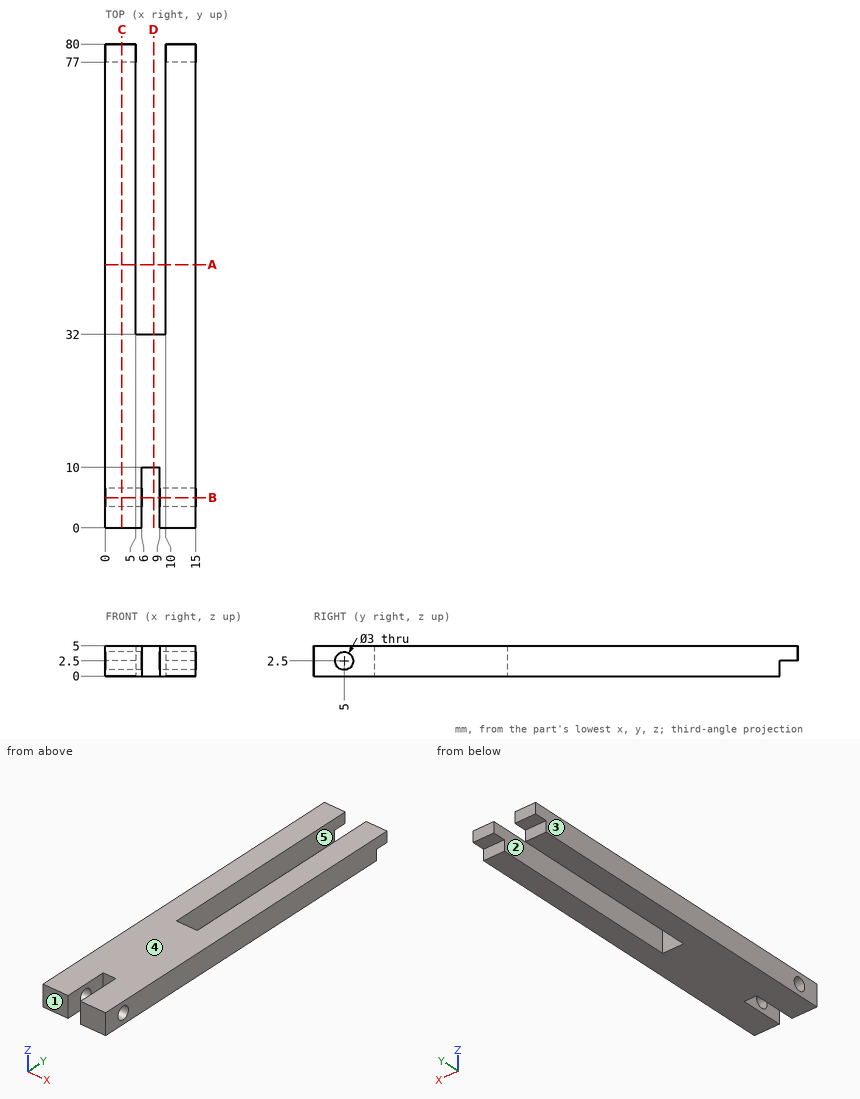
The drawing under review shows one solid part. Ordinate dimensions are in mm from its lowest x, y, z. A direction names the side the tool comes from. Coordinates: 2 decimals unless noted, no trailing zeros. Loops run counter-clockwise (first coordinate to the right, second up) from the corner with the lowest first, then second, coordinate; pieces in that order, holes last. Notation, with made-up numbers: M 23,47.5 L 66,47.5 A8 cw 66,53.5 Z; hole C -11,45 d9. An arc over 180 degrees is marked long. Use one line per item in the form item = value.
(1) Clearance check with flat-ended pins moving along their axes: P1, Ø1.5, axis at x = 13, y = 79, coming from the -Z side; P2, Ø2.5, axis at x = 7.5, z = 1.5, coming from the -Y side; P3, Ø0.8, axis at x = 3, z = 1, coming from the +Y side; P4, Ø1.8, axis at y = 5, z = 2.5, coming from the +X side. State where each tip first meets the part, or that it passes through.
Return value:
P1 = 2.5
P2 = 10
P3 = 77
P4 = through
(2) Consider section D-D (x = 8). Write out the cut boundary in (y, z), and give its area (3 significant figures).
Return value:
outline = M 10,0 L 32,0 L 32,5 L 10,5 Z
area = 110 mm2
(3) Draft analysis for pull direction X (two halves, no side actions). For the marked faces 3, 4 and 5, state which applies: pulls with the +X half, pulls with the -X half, needs draft (parallel to the pull), parting line crosses it, or undercut.
Return value:
face_3 = pulls with the -X half
face_4 = needs draft
face_5 = undercut
(4) Consider section C-C (x = 2.75). Write out the cut boundary in (y, z).
Return value:
outline = M 0,0 L 77,0 L 77,2.5 L 80,2.5 L 80,5 L 0,5 Z; hole C 5,2.5 d3
(5) Consider section A-A (y = 43.5). Write out the cut boundary in (x, z).
Return value:
outline = M 0,0 L 5,0 L 5,5 L 0,5 Z; M 10,0 L 15,0 L 15,5 L 10,5 Z
(6) Consider section B-B (y = 5). Write out the cut boundary in (x, z).
Return value:
outline = M 0,0 L 6,0 L 6,1 L 0,1 Z; M 0,4 L 6,4 L 6,5 L 0,5 Z; M 9,0 L 15,0 L 15,1 L 9,1 Z; M 9,4 L 15,4 L 15,5 L 9,5 Z
(7) For the marked faces 1 and 2, list the 3-axis set-ups (+Z, -Z, +X, -X, +Y, -Y) from which the entire face can be reached by the end or side of a thin tool; tool diameter is ignored.
Return value:
face_1 = +Z, -Z, +X, -X, -Y
face_2 = +Z, -Z, +Y
(8) For line 1 along X through (y, z) = (62.5, 4.45); line 2 along Z through (x, y) = (12.6, 5); line 3 along Y through (x, z) = (7.75, 1.1), list the stretches that pass through material, from the lowest coordinate up. Write a range as from..to.
Return value:
line_1 = 0..5, 10..15
line_2 = 0..1, 4..5
line_3 = 10..32
